Read the model definition and answer for the solid it produces. Units are mm, in the model's axes. Coordinates: 2 decimals unless noted, no trailing zeros. Order: outer loops, then holes, each group sorted by start corner. A loop starts at its lowest first (then second) coordinate and runs counter-clockwise, first axis right, second up. Notation, with made-up numbers: (75.25, 59.25) -> (111.25, 59.25) arc R16 ccw to (111.25, 63.25) -> close; hole circle Ø10 at (59.25, 25). An arc over 180 degrees is marked (long way). Answer as a JSON object with one key per item and string values. Group by question number.
1) Section C-C on y = -5.5 is taken. Determine the outline of the cut face in (x, z), and give its area (3 significant figures).
2) Given pin 1 (12.5 mm diameter, centred on y = -147.5, z = 810, fed in from +X); pin 2 (5 mm diameter, centred on y = 228, z = 285.5, fed in from +X), each flat-ended and moving along its own axis, determine where each tip first touches the part or whether it passes through.
3) Section A-A on x = 197 is taken. Count the separate pieces of the cut face and the enclosed holes in it, and give its area (3 significant figures).
4) Consider L1, parallel to X at y = -189, z = 234. Determine where the line is inside the solid, lowest interval first.
5) Section D-D on z = 251.5 is taken. Determine the outline of the cut face in (x, y).
from build123d import *

# Parameters (mm, degrees)
F0_W        = 370
F0_H        = 600
F1_DEPTH    = 800
F2_W        = 600
F2_H        = 80
F3_DEPTH    = 25
F5_DEPTH    = 50
F6_T1_DEPTH = 120
F6_T4_ANGLE = 180
F6_T6_ANGLE = 180
F7_W        = 40
F7_H        = 110
F8_DEPTH    = 25
F9_R        = 4.99999
F10_W       = 400
F10_H       = 600
F11_DEPTH   = 25


# Not quite as in the source:
# - a fillet or chamfer that OpenCascade refuses, or shapes differently, is made with other operations: its cross-section is extruded or revolved along the edge and cut away or added
# - a fillet or chamfer is up to 0.001 mm smaller than in the source, because OpenCascade refuses the exact size


with BuildPart() as f1:
    # F0 (on Top) → F1 (new body)
    with BuildSketch(Plane.XY):
        Rectangle(F0_W, F0_H)
    extrude(amount=F1_DEPTH)

    # F2 (on face) → F3 (cut)
    with BuildSketch(Plane.YZ.offset(185)):
        with Locations((0, 40)):
            Rectangle(F2_W, F2_H)
    extrude(amount=-F3_DEPTH, mode=Mode.SUBTRACT)

    # F4 (on face) → F5 (join)
    with BuildSketch(Plane.YZ.offset(185)):
        with BuildLine():
            ThreePointArc((-248.5795542598, 750), (-252.1150881657, 748.5355339059), (-253.5795542598, 745))
            Line((-253.5795542598, 745), (-253.5795542598, 625))
            ThreePointArc((-253.5795542598, 625), (-252.1150881657, 621.4644660941), (-248.5795542598, 620))
            ThreePointArc((-248.5795542598, 620), (-245.0440203538, 621.4644660941), (-243.5795542598, 625))
            Line((-243.5795542598, 625), (-243.5795542598, 745))
            ThreePointArc((-243.5795542598, 745), (-245.0440203538, 748.5355339059), (-248.5795542598, 750))
        make_face()
    extrude(amount=F5_DEPTH)

    # F6: fillet of radius 5 on 4 edges, made by hand

    # F6_s2 → F6_t1 (cut)
    with BuildSketch(Plane.XY.offset(625)):
        with BuildLine():
            ThreePointArc((230, -253.5795542598), (233.5355339059, -252.1150881657), (235, -248.5795542598))
            Line((235, -248.5795542598), (235, -253.5795542598))
            Line((235, -253.5795542598), (230, -253.5795542598))
        make_face()
        with BuildLine():
            ThreePointArc((230, -243.5795542598), (233.5355339059, -245.0440203538), (235, -248.5795542598))
            Line((235, -248.5795542598), (235, -243.5795542598))
            Line((235, -243.5795542598), (230, -243.5795542598))
        make_face()
    extrude(amount=F6_T1_DEPTH, mode=Mode.SUBTRACT)

    # F6_s3 → F6_t4 (revolve, cut)
    with BuildSketch(Plane.XY.offset(745)):
        with BuildLine():
            ThreePointArc((230, -253.5795542598), (233.5355339059, -252.1150881657), (235, -248.5795542598))
            Line((235, -248.5795542598), (235, -253.5795542598))
            Line((235, -253.5795542598), (230, -253.5795542598))
        make_face()
    revolve(axis=Axis((235, -248.5795542598, 745), (-1, 0, 0)), revolution_arc=F6_T4_ANGLE, mode=Mode.SUBTRACT)

    # F6_s5 → F6_t6 (revolve, cut)
    with BuildSketch(Plane.XY.offset(625)):
        with BuildLine():
            ThreePointArc((230, -243.5795542598), (233.5355339059, -245.0440203538), (235, -248.5795542598))
            Line((235, -248.5795542598), (235, -243.5795542598))
            Line((235, -243.5795542598), (230, -243.5795542598))
        make_face()
    revolve(axis=Axis((235, -248.5795542598, 625), (-1, 0, 0)), revolution_arc=F6_T6_ANGLE, mode=Mode.SUBTRACT)

    # F7 (on face) → F8 (cut)
    with BuildSketch(Plane(origin=(0, -243.5795542598, 0), x_dir=(-1, 0, 0), z_dir=(0, 1, 0))):
        with Locations((-205, 685)):
            Rectangle(F7_W, F7_H)
    extrude(amount=-F8_DEPTH, mode=Mode.SUBTRACT)

    # F9 (radius 5 in the source; OpenCascade refuses exactly that, so slightly less here)
    f9_edges = [f1.edges().sort_by_distance(p)[0] for p in [
        (205, -243.579554, 740),
        (225, -243.579554, 685),
        (205, -243.579554, 630),
        (205, -253.579554, 740),
        (225, -253.579554, 685),
        (205, -253.579554, 630),
    ]]
    fillet(f9_edges, radius=F9_R)

    # F10 (on face) → F11 (join)
    with BuildSketch(Plane.XY.offset(800)):
        with Locations((15, 0)):
            Rectangle(F10_W, F10_H)
    extrude(amount=F11_DEPTH)


solid = f1.part
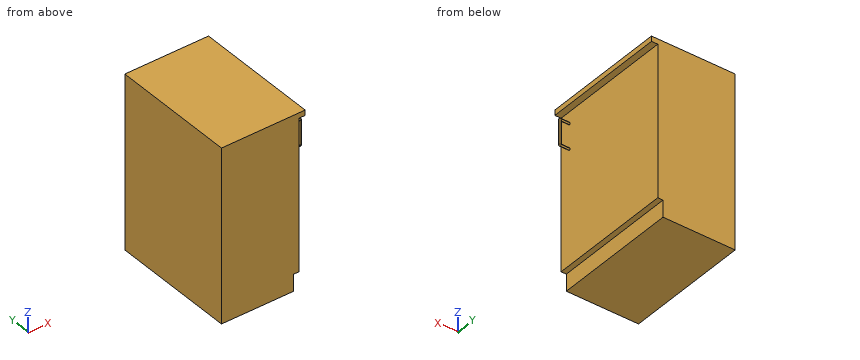
Worked answers:
{
 "1": {"outline": "(-185, 0) -> (160, 0) -> (160, 80) -> (185, 80) -> (185, 800) -> (215, 800) -> (215, 825) -> (-185, 825) -> close", "area": "304,000 mm²"},
 "2": {"pin 1": "stops at x = 215", "pin 2": "stops at x = 185"},
 "3": {"separate pieces": "3", "enclosed holes": "0", "area": "15,200 mm²"},
 "4": {"L1": "x = -185 to 185"},
 "5": {"outline": "(-185, -300) -> (185, -300) -> (185, 300) -> (-185, 300) -> close"}
}
